Build history of the part. All positions in model axes, mm. Face numbers are marked on the shaded views. Coordinates: 2 decimals unless noted, no trailing zeros. Loops run counter-clockwise (first coordinate to the right, second up) from the corner with the lowest first, then second, coordinate; pieces in that order, holes last.
(1) Slice it at B-B (z = 0). Give the cut face in (x, y), and give its area (3 significant figures).
(2) Slice it at C-C (x = 2.75). Give the cut face in (y, z).
(3) Two-plate mould, pull along Z, no slides. Class the marked faces 1, 2, 3 and 4: pulls with the +Z half, pulls with the -Z half, needs draft (parallel to the pull), parting line crosses it, or undercut.
(4) Slice it at D-D (z = 3.5). Give the cut face in (x, y), and give its area (3 significant figures).
(5) Flat gauge pins, fed straight in: P1, Ø3, axis at y = 3, z = 3.5, coming from the +X side; P2, Ø1.5, axis at y = 5, z = -2.5, coming from the +X side; P3, Ø1.5, axis at x = 0, y = 4, coming from the +Z side. Where does each tip first touch, or does it go through?
(6) Slice it at A-A (x = -0.25). Give the cut face in (y, z).
(7) Wall check: L1, parallel to Y at x = 3, z = -3.25; L2, parallel to Z at x = -1.5, y = 4.25; L3, parallel to Z at x = -0.5, y = 5.5. Give the ranges that are in metal, low to high.
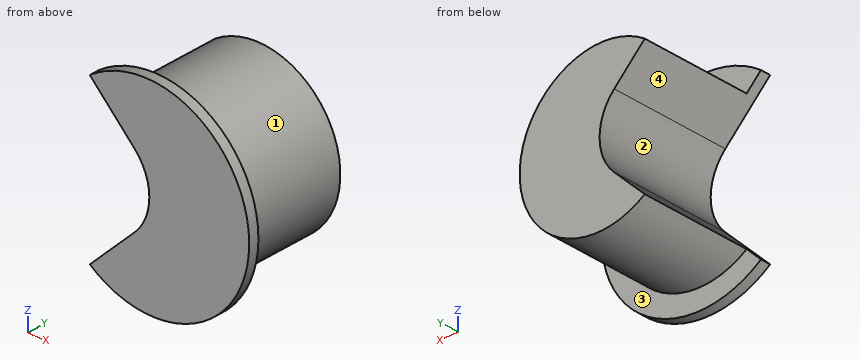
from build123d import *

# Parameters (mm, degrees)
SKETCH1_R           = 5
SKETCH1_R_2         = 4
BOSS_EXTRUDE1_DEPTH = 0.5
SKETCH1_3_R         = 4
BOSS_EXTRUDE2_DEPTH = 6
CUT_EXTRUDE2_DEPTH  = 10.273618495


with BuildPart() as part:
    # Sketch1 → Boss-Extrude1 (new body)
    with BuildSketch(Plane(origin=(0, 0, 0), x_dir=(1, 0, 0), z_dir=(0, 1, 0))):
        with Locations(Location((0, 0, 0), (0, 0, 270))):
            Circle(SKETCH1_R)
        with Locations(Location((0, 0, 0), (0, 0, 270))):
            Circle(SKETCH1_R_2, mode=Mode.SUBTRACT)
    extrude(amount=BOSS_EXTRUDE1_DEPTH)

    # Sketch1_3 → Boss-Extrude2 (add)
    with BuildSketch(Plane(origin=(0, 0, 0), x_dir=(1, 0, 0), z_dir=(0, 1, 0))):
        with Locations(Location((0, 0, 0), (0, 0, 270))):
            Circle(SKETCH1_3_R)
    extrude(amount=BOSS_EXTRUDE2_DEPTH)

    # Sketch2 → Cut-Extrude2 (cut, through all)
    with BuildSketch(Plane(origin=(0, 0, 0), x_dir=(1, 0, 0), z_dir=(0, 1, 0))):
        with BuildLine():
            Line((-0.732233047, 1.767766953), (-2.979648862, 4.015182768))
            ThreePointArc((-2.979648862, 4.015182768), (-5, 0), (-2.979648862, -4.015182768))
            Line((-2.979648862, -4.015182768), (-0.732233047, -1.767766953))
            ThreePointArc((-0.732233047, -1.767766953), (0, 0), (-0.732233047, 1.767766953))
        make_face()
    extrude(amount=CUT_EXTRUDE2_DEPTH, mode=Mode.SUBTRACT)


solid = part.part
Response values:
1. outline: (0, 0) - (5, 0) - (5, 0.5) - (4, 0.5) - (4, 6) - (0, 6) - close
1. area: 24.5 mm2
2. outline: (0, -4.18) - (0.5, -4.18) - (0.5, -2.9) - (6, -2.9) - (6, 2.9) - (0.5, 2.9) - (0.5, 4.18) - (0, 4.18) - close
3. face 1: parting line crosses it
3. face 2: undercut
3. face 3: needs draft
3. face 4: undercut
4. outline: (-2.46, 0) - (3.57, 0) - (3.57, 0.5) - (1.94, 0.5) - (1.94, 6) - (-1.94, 6) - (-1.94, 0.5) - (-2.46, 0.5) - close
4. area: 24.3 mm2
5. P1: stops at x = 3.46
5. P2: stops at x = 3.6
5. P3: stops at z = 4
6. outline: (0, -4.99) - (0.5, -4.99) - (0.5, -3.99) - (6, -3.99) - (6, -1.09) - (0, -1.09) - close; (0, 1.09) - (6, 1.09) - (6, 3.99) - (0.5, 3.99) - (0.5, 4.99) - (0, 4.99) - close
7. L1: y = 0 to 0.5
7. L2: z = -3.71 to -2.54, 2.54 to 3.71
7. L3: z = -3.97 to -1.5, 1.5 to 3.97
